```python
from build123d import *

# Parameters (mm, degrees)
F0_W     = 1.35
F0_H     = 50
F1_DEPTH = 500


with BuildPart() as f1:
    # F0 (on Front) → F1 (new body)
    with BuildSketch(Plane.XZ):
        Polygon((0, 1), (56.25, 1), (56.25, 3.5), (55.75, 3.5), (55.75, 53.5), (54.4, 53.5), (54.4, 3.5), (50.75, 3.5), (49.4, 3.5), (45.75, 3.5), (44.4, 3.5), (40.75, 3.5), (39.4, 3.5), (35.75, 3.5), (34.4, 3.5), (30.75, 3.5), (29.4, 3.5), (25.75, 3.5), (24.4, 3.5), (20.75, 3.5), (19.4, 3.5), (15.75, 3.5), (14.4, 3.5), (10.75, 3.5), (9.4, 3.5), (5.75, 3.5), (4.4, 3.5), (0.75, 3.5), (-0.6, 3.5), (-4.25, 3.5), (-5.6, 3.5), (-9.25, 3.5), (-10.6, 3.5), (-14.25, 3.5), (-15.6, 3.5), (-19.25, 3.5), (-20.6, 3.5), (-24.25, 3.5), (-25.6, 3.5), (-29.25, 3.5), (-30.6, 3.5), (-34.25, 3.5), (-35.6, 3.5), (-39.25, 3.5), (-40.6, 3.5), (-44.25, 3.5), (-45.6, 3.5), (-49.25, 3.5), (-50.6, 3.5), (-52.25, 3.5), (-54.25, 3.5), (-55.6, 3.5), (-56.25, 3.5), (-56.25, 1), align=None)
        with Locations((-54.925, 28.5)):
            Rectangle(F0_W, F0_H)
        with Locations((50.075, 28.5)):
            Rectangle(F0_W, F0_H)
        with Locations((-49.925, 28.5)):
            Rectangle(F0_W, F0_H)
        with Locations((45.075, 28.5)):
            Rectangle(F0_W, F0_H)
        with Locations((-44.925, 28.5)):
            Rectangle(F0_W, F0_H)
        with Locations((40.075, 28.5)):
            Rectangle(F0_W, F0_H)
        with Locations((-39.925, 28.5)):
            Rectangle(F0_W, F0_H)
        with Locations((35.075, 28.5)):
            Rectangle(F0_W, F0_H)
        with Locations((-34.925, 28.5)):
            Rectangle(F0_W, F0_H)
        with Locations((30.075, 28.5)):
            Rectangle(F0_W, F0_H)
        with Locations((-29.925, 28.5)):
            Rectangle(F0_W, F0_H)
        with Locations((25.075, 28.5)):
            Rectangle(F0_W, F0_H)
        with Locations((-24.925, 28.5)):
            Rectangle(F0_W, F0_H)
        with Locations((20.075, 28.5)):
            Rectangle(F0_W, F0_H)
        with Locations((-19.925, 28.5)):
            Rectangle(F0_W, F0_H)
        with Locations((15.075, 28.5)):
            Rectangle(F0_W, F0_H)
        with Locations((-14.925, 28.5)):
            Rectangle(F0_W, F0_H)
        with Locations((10.075, 28.5)):
            Rectangle(F0_W, F0_H)
        with Locations((-9.925, 28.5)):
            Rectangle(F0_W, F0_H)
        with Locations((5.075, 28.5)):
            Rectangle(F0_W, F0_H)
        with Locations((-4.925, 28.5)):
            Rectangle(F0_W, F0_H)
        with Locations((0.075, 28.5)):
            Rectangle(F0_W, F0_H)
    extrude(amount=F1_DEPTH)


solid = f1.part
```
Geometry check sheet. Reference: the model listing, model coordinates, mm. A direction names the side the tool comes from. Give positions to 0.01 mm unless a question says otherwise; leave off trailing zeros. Write item = value, one per line. Start each with the question number.
1. Section check A-A, the plane z = 24.5. Give the number of separate pieces and of enclosed holes in the cut face, plus the area to 3 significant figures.
2. Go/stop test with flat-tipped pins: P1, Ø15, axis at y = -283.5, z = 39, coming from the -X side; P2, Ø1.8, axis at x = 7, y = -205, coming from the +Z side; P3, Ø1.5, axis at y = -379.5, z = 19.5, coming from the +X side. Record where each tip stops, or that it passes through.
3. Thickness scan on probe 1 along Z at (x, y) = (-48.5, -270). Record the ranges inside material, lowest first.
4. Tool access check on faces 5 (the face through (-4.4, 0, 25.4)), 6 (the face through (25.75, -246, 28)). Record the directions out of +Z, -Z, +X, -X, +Y, -Y that give a thin tool (end or side, any length) a straight path to the whole face; none if there is none.
5. Draft check along X on faces 1 (the face through (55.75, -246, 28)), 2 (the face through (49.4, -246, 28)), 3 (the face through (-55.6, -246, 28)), 4 (the face through (35.75, -246, 28)). Enter one of: +X half, -X half, draft (parallel to the pull), parting line (faces both ways), or undercut.
Values follow:
q1.separate_pieces = 23
q1.enclosed_holes = 0
q1.area = 15,500 mm^2
q2.P1 = -55.6
q2.P2 = 3.5
q2.P3 = 55.75
q3.probe_1 = 1 to 3.5
q4.face_5 = +Z, -Z, +X, -X, +Y
q4.face_6 = +Z, +Y, -Y
q5.face_1 = +X half
q5.face_2 = undercut
q5.face_3 = -X half
q5.face_4 = undercut
